Work out the finished part from the listing and answer in its coordinate system (mm). A direction names the side the tool comes from. Give positions to 0.01 mm unless a question says otherwise; leave off trailing zeros. Write each loop counter-clockwise with the first axis right and the second up, starting at its lowest first coordinate (ties: lowest second). Pieces come first, ordered by that corner, then holes.
1) A tool of negligible diameter and unlimited length cuts with its end or side. For faces 4 (the face through (0, -6, 114.2)), 5 (the face through (10, -2, 58)), 6 (the face through (5, 5, 108.6)), from which of +Z, -Z, +X, -X, +Y, -Y can it reach the whole face along a straight path? Write none if from no direction.
2) Straight lines are drawn through the part: probe 1 along Z at (x, y) = (-4.75, -4.5); probe 2 along Z at (x, y) = (3.25, 8.5); probe 3 along Y at (x, z) = (7, 101). For each, find the intervals that lie inside material, in ascending order.
3) Find section A-A (y = -5.25). Determine the outline of the cut face in (x, z), plus the area to 3 significant figures.
4) Given pin 1 Ø1 at (y, z) = (5.5, 16.5) entering from +X; pin 2 Ø5 at (x, z) = (5.5, 66) entering from +Y, each flat-ended and moving along its own axis, determine where each tip first touches the part or whether it passes through.
5) Find section D-D (y = 1). Determine the outline of the cut face in (x, z).
6) Find section B-B (x = 7.25). Determine the outline of the cut face in (y, z).
7) Determine the mould class of faces 1 (the face through (0, -3.5, 6)), 2 (the face through (0, 0, 0)), 3 (the face through (0, -10, 58)) for opening direction Y: pulls with the +Y half, pulls with the -Y half, needs draft (parallel to the pull), parting line crosses it, or undercut.
8) Find section C-C (z = 74.5). Determine the outline of the cut face in (x, y), plus the area to 3 significant figures.
```python
from build123d import *

# Parameters (mm, degrees)
BOX_W        = 40
BOX_H        = 40
BOX_DEPTH    = 98.6
BOX001_W     = 20
BOX001_H     = 20
BOX001_DEPTH = 118.6
SKETCH_W     = 4
SKETCH_H     = 4
POCKET_DEPTH = 30


with BuildPart() as battery_hole:
    # Box → Box (new body)
    with BuildSketch(Plane.XY.offset(10)):
        with Locations((20, 20)):
            Rectangle(BOX_W, BOX_H)
    extrude(amount=BOX_DEPTH)


with BuildPart() as pocket:
    # Box001 → Box001 (new body)
    with BuildSketch(Plane(origin=(-10, -10, 0), x_dir=(1, 0, 0), z_dir=(0, 0, 1))):
        with Locations((10, 10)):
            Rectangle(BOX001_W, BOX001_H)
    extrude(amount=BOX001_DEPTH)

    # Cut: cut Battery Hole
    add(battery_hole.part, mode=Mode.SUBTRACT)

    # Sketch → Pocket (cut)
    with BuildSketch(Plane.YZ.offset(10)):
        with Locations((-5.5, 112.2)):
            Rectangle(SKETCH_W, SKETCH_H)
        with Locations((-5.5, 6.2)):
            Rectangle(SKETCH_W, SKETCH_H)
    extrude(amount=-POCKET_DEPTH, mode=Mode.SUBTRACT)


solid = pocket.part
```
Results:
1. face 4: +X, -X
1. face 5: +Z, -Z, +X, +Y, -Y
1. face 6: +X, +Y
2. probe 1: z = 0 to 4.2, 8.2 to 110.2, 114.2 to 118.6
2. probe 2: z = 0 to 10, 108.6 to 118.6
2. probe 3: y = -10 to 0
3. outline: (-10, 0) - (10, 0) - (10, 4.2) - (-10, 4.2) - close; (-10, 8.2) - (10, 8.2) - (10, 110.2) - (-10, 110.2) - close; (-10, 114.2) - (10, 114.2) - (10, 118.6) - (-10, 118.6) - close
3. area: 2,210 mm2
4. pin 1: stops at x = 0
4. pin 2: stops at y = 0
5. outline: (-10, 0) - (10, 0) - (10, 10) - (0, 10) - (0, 108.6) - (10, 108.6) - (10, 118.6) - (-10, 118.6) - close
6. outline: (-10, 0) - (10, 0) - (10, 10) - (0, 10) - (0, 108.6) - (10, 108.6) - (10, 118.6) - (-10, 118.6) - close; hole (-7.5, 4.2) - (-3.5, 4.2) - (-3.5, 8.2) - (-7.5, 8.2) - close; hole (-7.5, 110.2) - (-3.5, 110.2) - (-3.5, 114.2) - (-7.5, 114.2) - close
7. face 1: undercut
7. face 2: needs draft
7. face 3: pulls with the -Y half
8. outline: (-10, -10) - (10, -10) - (10, 0) - (0, 0) - (0, 10) - (-10, 10) - close
8. area: 300 mm2
